from build123d import *

# Parameters (mm, degrees)
F0_W     = 30
F0_H     = 10.9
F0_W_2   = 6.35
F1_DEPTH = 3.175
F2_DEPTH = 6.35
F3_R     = 3.175
F4_R     = 3.175
F5_R     = 1.5875


with BuildPart() as f1:
    # F0 (on Top) → F1 (new body)
    with BuildSketch(Plane.XY):
        Polygon((-15, 5.45), (15, 5.45), (15, -5.45), (-15, -5.45), (-21.35, -5.45), (-21.35, -11.8), (21.35, -11.8), (21.35, 11.8), (-21.35, 11.8), (-21.35, 5.45), align=None)
        Rectangle(F0_W, F0_H)
        with Locations((-18.175, 0)):
            Rectangle(F0_W_2, F0_H)
    extrude(amount=-F1_DEPTH)

    # F0 (on Top) → F2 (join)
    with BuildSketch(Plane.XY):
        Polygon((-15, 5.45), (15, 5.45), (15, -5.45), (-15, -5.45), (-21.35, -5.45), (-21.35, -11.8), (21.35, -11.8), (21.35, 11.8), (-21.35, 11.8), (-21.35, 5.45), align=None)
    extrude(amount=F2_DEPTH)

    # F3
    f3_edges = [f1.edges().sort_by_distance(p)[0] for p in [
        (-21.35, 5.45, 3.175),
        (-21.35, -5.45, 3.175),
    ]]
    fillet(f3_edges, radius=F3_R)

    # F4
    f4_edges = [f1.edges().sort_by_distance(p)[0] for p in [
        (-1.5875, 5.45, 6.35),
        (-1.5875, -5.45, 6.35),
        (15, 0, 6.35),
    ]]
    fillet(f4_edges, radius=F4_R)

    # F5
    f5_edges = [f1.edges().sort_by_distance(p)[0] for p in [
        (0, -11.8, -3.175),
        (21.35, 0, -3.175),
        (0, 11.8, -3.175),
        (-21.35, 0, -3.175),
    ]]
    fillet(f5_edges, radius=F5_R)


solid = f1.part
Work out the finished part from the listing and answer in its coordinate system (mm). A direction names the side the tool comes from. Coordinates: 2 decimals unless noted, no trailing zeros. Order: outer loops, then holes, each group sorted by start corner. A loop starts at its lowest first (then second) coordinate and runs counter-clockwise, first axis right, second up. Notation, with made-up numbers: (51.5, 26) - (96.5, 26) arc R23 cw to (96.5, 52) - close; hole circle Ø11 at (88, -23). An arc over 180 degrees is marked (long way). Put each result on its own line as item: value. Start each with the question number.
1) For a pull along Y with two mould halves and no side action, classify faces 3 (the cylindrical face through (-0.299, 11.347, -2.698)), 4 (the cylindrical face through (-20.4, 10.19, 5.44)), 5 (the flat face through (15, 0, 2)) as released by +Y, released by -Y, zero draft, split by the parting line, or undercut.
2) Find the intervals of material crossed by line 1 (Y direction, x = 13, z = 0.5); line 2 (X direction, y = -1, z = 0.5); line 3 (Y direction, x = 2, z = 4.75), in increasing order. Write a range as from..to.
3) For faces 1 (the cylindrical face through (0.299, -11.347, -2.698)), 2 (the flat face through (-1, -5.45, 2)), determine the directions among +Z, -Z, +X, -X, +Y, -Y from which every point of the face is accessible in a straight line to the end or side of a thin tool.
4) Flat-ended cylindrical pins translate along their axes: pin 1 (2.5 mm diameter, centred on y = 2, z = 1.5, fed in from -X); pin 2 (1.5 mm diameter, centred on x = -8.5, y = 0.5, fed in from +Z). Find the tip coordinate at first contact, or state that the pin passes through.
5) Find section C-C (z = 5). Give the vertices of the cut face in (x, y) (3 decimals), plus the area to 3 significant figures.
Results list:
1. face 3: released by +Y
1. face 4: zero draft
1. face 5: undercut
2. line 1: y = -11.8..-5.45, 5.45..11.8
2. line 2: x = 15..21.35
2. line 3: y = -11.8..-5.87, 5.87..11.8
3. face 1: -Z, +X, -X, -Y
3. face 2: +Z, -X
4. pin 1: stops at x = 15
4. pin 2: stops at z = 0
5. outline: (-20.773, -11.8) - (21.35, -11.8) - (21.35, 11.8) - (-20.773, 11.8) - (-20.773, 8.625) arc R2.598 ccw to (-18.175, 6.027) - (15.577, 6.027) - (15.577, -6.027) - (-18.175, -6.027) arc R2.598 ccw to (-20.773, -8.625) - close
5. area: 553 mm^2
